```python
from build123d import *

# Parameters (mm, degrees)
F0_W     = 200
F0_H     = 100
F1_DEPTH = 8
F2_W     = 200
F2_H     = 100
F2_R     = 30
F3_DEPTH = 2
F4_W     = 200
F4_H     = 100
F4_R     = 30
F5_DEPTH = 5
F6_R     = 45
F6_R_2   = 5
F6_R_3   = 30
F7_DEPTH = 5
F8_DEPTH = 5


with BuildPart() as f1:
    # F0 (on Top) → F1 (new body)
    with BuildSketch(Plane.XY):
        Rectangle(F0_W, F0_H)
    extrude(amount=F1_DEPTH)

    # F2 (on face) → F3 (join)
    with BuildSketch(Plane.XY.offset(8)):
        Rectangle(F2_W, F2_H)
        Circle(F2_R, mode=Mode.SUBTRACT)
    extrude(amount=F3_DEPTH)

    # F4 (on face) → F5 (join)
    with BuildSketch(Plane.XY.offset(10)):
        Rectangle(F4_W, F4_H)
        with BuildLine():
            ThreePointArc((-90, 28), (-86.4852813742, 36.4852813742), (-78, 40))
            Line((-78, 40), (-72, 40))
            ThreePointArc((-72, 40), (-63.5147186258, 36.4852813742), (-60, 28))
            Line((-60, 28), (-60, -28))
            ThreePointArc((-60, -28), (-63.5147186258, -36.4852813742), (-72, -40))
            Line((-72, -40), (-78, -40))
            ThreePointArc((-78, -40), (-86.4852813742, -36.4852813742), (-90, -28))
            Line((-90, -28), (-90, 28))
        make_face(mode=Mode.SUBTRACT)
        Circle(F4_R, mode=Mode.SUBTRACT)
    extrude(amount=F5_DEPTH)

    # F6 (on face) → F7 (join)
    with BuildSketch(Plane.XY.offset(15)):
        Circle(F6_R)
        with Locations((0, -37.5)):
            Circle(F6_R_2, mode=Mode.SUBTRACT)
        with Locations((-37.5, 0)):
            Circle(F6_R_2, mode=Mode.SUBTRACT)
        Circle(F6_R_3, mode=Mode.SUBTRACT)
        with Locations((37.5, 0)):
            Circle(F6_R_2, mode=Mode.SUBTRACT)
        with Locations((0, 37.5)):
            Circle(F6_R_2, mode=Mode.SUBTRACT)
    extrude(amount=F7_DEPTH)

    # F8 (add): a face of the model
    f8_faces = [f1.faces().sort_by_distance(p)[0] for p in [
        (97.7639320225, 0, 15),
    ]]
    extrude(f8_faces, amount=F8_DEPTH)


solid = f1.part
```
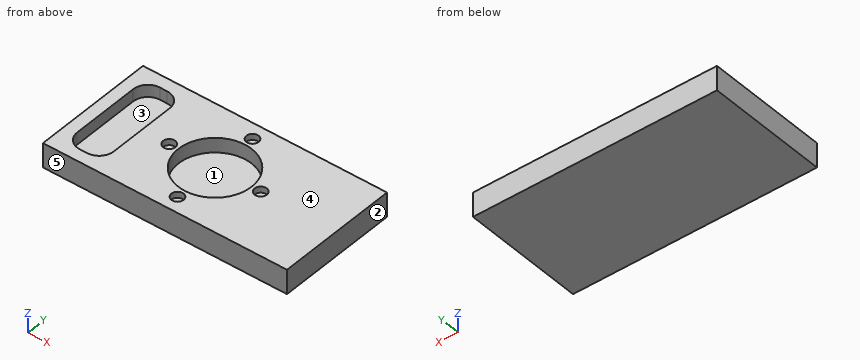
Geometry check sheet. Reference: the model listing, model coordinates, mm. Face numbers are marked on the shaded views. A direction names the side the tool comes from. Coordinates: 2 decimals unless noted, no trailing zeros. Order: outer loops, then holes, each group sorted by start corner. A loop starts at its lowest first (then second) coordinate and runs counter-clockwise, first axis right, second up. Notation, with made-up numbers: M -19.75,-30.5 L 34.25,-30.5 A24 ccw 34.25,4.5 Z; hole C 12.25,27.25 d4. An arc over 180 degrees is marked long. Answer as a JSON object with one key per item and string values.
Q1. Cross-section at B-B on x = 0. Record the cut outline in (y, z).
Results are:
{"outline": "M -50,0 L 50,0 L 50,20 L 42.5,20 L 42.5,15 L 32.5,15 L 32.5,20 L 30,20 L 30,8 L -30,8 L -30,20 L -32.5,20 L -32.5,15 L -42.5,15 L -42.5,20 L -50,20 Z"}
Q2. Cross-section at D-D on y = 19.5. Record the cut outline in (x, z), and give its area (3 significant figures).
Results are:
{"outline": "M -100,0 L 100,0 L 100,20 L 22.8,20 L 22.8,8 L -22.8,8 L -22.8,20 L -60,20 L -60,10 L -90,10 L -90,20 L -100,20 Z", "area": "3,150 mm²"}
Q3. Tool access check on the marked faces 1 and 2. Record the directions out of +Z, -Z, +X, -X, +Y, -Y that give a thin tool (end or side, any length) a straight path to the whole face; none if there is none.
Results are:
{"face 1": "+Z", "face 2": "+Z, -Z, +X, +Y, -Y"}
Q4. Cross-section at C-C on x = -37.5. Record the cut outline in (y, z), and give its area (3 significant figures).
Results are:
{"outline": "M -50,0 L 50,0 L 50,20 L 5,20 L 5,15 L -5,15 L -5,20 L -50,20 Z", "area": "1,950 mm²"}
Q5. Scan lines: line 1 (Y direction, x = 0, z = 18.3); line 2 (Y direction, x = -37.5, z = 17.55); line 3 (X direction, y = 2, z = 11.25). Record each from-to range of solid material in increasing order.
Results are:
{"line 1": "y = -50 to -42.5, -32.5 to -30, 30 to 32.5, 42.5 to 50", "line 2": "y = -50 to -5, 5 to 50", "line 3": "x = -100 to -90, -60 to -29.93, 29.93 to 100"}
Q6. Cross-section at A-A on y = 0. Record the cut outline in (x, z).
Results are:
{"outline": "M -100,0 L 100,0 L 100,20 L 42.5,20 L 42.5,15 L 32.5,15 L 32.5,20 L 30,20 L 30,8 L -30,8 L -30,20 L -32.5,20 L -32.5,15 L -42.5,15 L -42.5,20 L -60,20 L -60,10 L -90,10 L -90,20 L -100,20 Z"}
Q7. Depth check by flat-ended pin: pin 1 Ø5 at (x, y) = (1.5, -37.5) entering from +Z; pin 2 Ø18 at (x, y) = (2, -10.5) entering from +Z; pin 3 Ø1 at (x, y) = (-76, -5) entering from +Z. Enter the tip coordinate at first touch or a pass-through.
Results are:
{"pin 1": "stops at z = 15", "pin 2": "stops at z = 8", "pin 3": "stops at z = 10"}
Q8. Release check for a two-part mould opening along Y. For the marked faces 3, 4 and 5 record: released by +Y, released by -Y, zero draft, split by the parting line, or undercut.
Results are:
{"face 3": "undercut", "face 4": "zero draft", "face 5": "released by -Y"}
